Read the model definition and answer for the solid it produces. Units are mm, in the model's axes. A direction names the side the tool comes from. Round coordinates to 2 decimals unless told otherwise and drop trailing zeros. Loops run counter-clockwise (first coordinate to the right, second up) from the corner with the lowest first, then second, coordinate; pieces in that order, holes last. Notation, with made-up numbers: M 61.5,66 L 106.5,66 A18 ccw 106.5,96 Z; hole C -9,-18.75 d8. An arc over 180 degrees is marked long. Answer as CSV lines item,"result".
```python
from build123d import *

# Parameters (mm, degrees)
ENL_V_START                  = -1
ENL_V_MAT_EXTRU_1_DEPTH      = 7
R_P_TITION_CIRCULAIRE1_COUNT = 6


with BuildPart() as part:
    # Esquisse2 → Révolution1 (revolve)
    with BuildSketch(Plane.XY, mode=Mode.PRIVATE) as r_volution1_sk:
        with BuildLine():
            Line((4.5, 0), (7.201056776, 0))
            ThreePointArc((7.201056776, 0), (9.766863159, 0.70853899), (11.605479997, 2.633344958))
            Line((11.605479997, 2.633344958), (12.75, 4.763334496))
            Line((12.75, 4.763334496), (12.309557678, 5))
            Line((12.309557678, 5), (11.023538577, 2.606675967))
            ThreePointArc((11.023538577, 2.606675967), (9.552645106, 1.066831192), (7.5, 0.5))
            Line((7.5, 0.5), (4.5, 0.5))
            Line((4.5, 0.5), (4.5, 0))
        make_face()
    revolve(r_volution1_sk.sketch.rotate(Axis((0, 0, 0), (0, 1, 0)), 90), axis=Axis((0, 0, 0), (0, 1, 0)))  # turned: the seam where the file's is

    # Esquisse3 → Enlèv. mat.-Extru.1 (cut)
    with BuildSketch(Plane(origin=(0, 0, 0), x_dir=(1, 0, 0), z_dir=(0, 1, 0)).offset(ENL_V_START)):
        with BuildLine():
            Line((-49.624128755, 62.90410991), (-2.5, 12.50249975))
            Line((-2.5, 12.50249975), (-0.584366138, 10.453633624))
            ThreePointArc((-0.584366138, 10.453633624), (0, 10.2), (0.584366138, 10.453633624))
            Line((0.584366138, 10.453633624), (2.5, 12.50249975))
            Line((2.5, 12.50249975), (49.624128755, 62.90410991))
            Line((49.624128755, 62.90410991), (49.624128755, 200.904194224))
            Line((49.624128755, 200.904194224), (-49.624128755, 200.904194224))
            Line((-49.624128755, 200.904194224), (-49.624128755, 62.90410991))
        make_face()
    enl_v_mat_extru_1 = extrude(amount=ENL_V_MAT_EXTRU_1_DEPTH, mode=Mode.SUBTRACT)

    # Répétition circulaire1: Enlèv. mat.-Extru.1 ×6 about axis
    r_p_tition_circulaire1_axis = Axis((0, 0, 0), (0, 1, 0))
    for i in range(1, R_P_TITION_CIRCULAIRE1_COUNT):
        add(enl_v_mat_extru_1.rotate(r_p_tition_circulaire1_axis, i * 360 / R_P_TITION_CIRCULAIRE1_COUNT), mode=Mode.SUBTRACT)


solid = part.part
```
1) Determine the mould class of faces 1 (the conical face through (12.48, 4.91, 0.06)), 2 (the flat face through (1.47, 3.1, -11.4)), 3 (the flat face through (5, 0.5, 0)), 4 (the conical face through (6.186, 4.91, 10.836)) for opening direction Z: released by +Z, released by -Z, zero draft, split by the parting line, or undercut.
Evaluation:
face 1,"split by the parting line"
face 2,"released by -Z"
face 3,"undercut"
face 4,"released by +Z"
2) Straight lines are drawn through the part: line 1 (Y direction, x = 2, z = -5); line 2 (X direction, y = 0.45, z = 0); line 3 (Z direction, x = -8.25, y = 3.3). For each, find the intervals that lie inside material, in ascending order.
Evaluation:
line 1,"y = 0 to 0.5"
line 2,"x = -9.27 to -4.5, 4.5 to 9.27"
line 3,"z = -8.66 to -7.86, 7.86 to 8.66"
3) Each of these flat-tipped pins is pushed along its axis until it touches: P1, Ø6, axis at x = -2.5, z = -1.5, coming from the +Y side; P2, Ø1, axis at y = 2, z = -3.5, coming from the +X side; P3, Ø3, axis at y = 3.5, z = -5, coming from the +X side; P4, Ø7, axis at x = 0, z = 0, coming from the -Y side. Where does it stop, or does it pass through?
Evaluation:
P1,"stops at y = 0.5"
P2,"stops at x = 11.02"
P3,"stops at x = 12.04"
P4,"passes through"
4) Find section A-A, the plane z = 0. Give the vertices of the cut face in (x, y).
Evaluation:
outline,"M -12.75,4.76 L -11.61,2.63 A5 ccw -7.2,0 L -4.5,0 L -4.5,0.5 L -7.5,0.5 A4 cw -11.02,2.61 L -12.31,5 Z; M 4.5,0 L 7.2,0 A5 ccw 11.61,2.63 L 12.75,4.76 L 12.31,5 L 11.02,2.61 A4 cw 7.5,0.5 L 4.5,0.5 Z"
5) A tool of negligible diameter and unlimited length cuts with its end or side. For faces 5 (the conical face through (-5.698, 3.521, -10.006)), 6 (the flat face through (-1.547, 3.24, -11.483)), 7 (the flat face through (9.137, 3.099, 6.969)), 8 (the flat face through (-9.137, 3.099, -6.969)), from which of +Z, -Z, +X, -X, +Y, -Y can it reach the whole face along a straight path? Write none if from no direction.
Evaluation:
face 5,"+Y"
face 6,"-Z, +Y, -Y"
face 7,"+X, +Y, -Y"
face 8,"-X, +Y, -Y"
6) Find section B-B, the plane x = 0. Give the vertices of the cut face in (y, z).
Evaluation:
outline,"M 0,-7.2 A5 ccw 1,-10.2 L 1.55,-10.2 A4 cw 0.5,-7.5 L 0.5,-4.5 L 0,-4.5 Z; M 0,4.5 L 0.5,4.5 L 0.5,7.5 A4 cw 1.55,10.2 L 1,10.2 A5 ccw 0,7.2 Z"
